Autodesk Inventor part; units mm, degrees
ref_plane "YZ Plane" through (0, 0, 0) normal (1, 0, 0) x (0, 1, 0)
ref_plane "XZ Plane" through (0, 0, 0) normal (0, 1, 0) x (-1, 0, 0)
ref_plane "XY Plane" through (0, 0, 0) normal (0, 0, 1) x (1, 0, 0)
sketch "Boceto1" plane through (0, 0, 0) normal (0, 1, 0) x (-1, 0, 0)
  line L0 (1.7308, 43.9183) -> (-63.2692, 43.9183)
  line L1 (-63.2692, 43.9183) -> (-63.2692, -61.0817)
  line L2 (-63.2692, -61.0817) -> (1.7308, -61.0817)
  line L3 (1.7308, -61.0817) -> (1.7308, 43.9183)
  point P0 (0, 0)
  dimension "d0" = 105
  dimension "d1" = 65
extrude "Extrusión1" add sketch "Boceto1" along normal blind 25
shell "Vaciado1" thickness 5 removed faces 1 at (19.9359, 25, -26.0817)
sketch "Boceto2" plane through (0, 25, 0) normal (0, 1, 0) x (1, 0, 0)
  line L0 (3.2692, 56.0817) -> (3.2692, -38.9183)
  line L1 (58.2692, 56.0817) -> (3.2692, 56.0817)
  line L2 (3.2692, 56.0817) -> (3.2692, -38.9183)
  line L3 (3.2692, -38.9183) -> (58.2692, -38.9183)
  line L4 (58.2692, -38.9183) -> (58.2692, 56.0817)
  point P0 (0, 0)
extrude "Extrusión2" add sketch "Boceto2" against normal blind 5
sketch "Boceto3" plane through (-1.7308, 0, 43.9183) normal (0, 0, 1) x (1, 0, 0)
  circle A0 centre (12.5, 12.5) radius 4.5
  line L0 (0, 0) -> (65, 0)
  line L1 (0, 0) -> (0, 25)
  point P0 (1.7308, 0)
  dimension "d12" = 9
  dimension "d13" = 12.5
  dimension "d14" = 12.5
extrude "Extrusión3" cut sketch "Boceto3" against normal blind 5
sketch "Boceto4" plane through (-1.7308, 0, 43.9183) normal (0, 0, 1) x (1, 0, 0)
  line L0 (60, 20) -> (5, 20)
  line L1 (60, 5) -> (5, 5)
  line L2 (29.5, 20) -> (35.5, 20)
  line L3 (35.5, 20) -> (35.5, 5)
  line L4 (35.5, 5) -> (29.5, 5)
  line L5 (29.5, 5) -> (29.5, 20)
  line L6 (0, 0) -> (0, 25)
  line L7 (65, 0) -> (65, 25)
  point P0 (1.7308, 0)
  point P1 (29.5, 12.5)
  point P2 (0, 12.5)
  dimension "d17" = 6
  dimension "d18" = 29.5
  dimension "d19" = 29.5
extrude "Extrusión4" cut sketch "Boceto4" against normal blind 5
sketch "Boceto5" plane through (-1.7308, 0, 43.9183) normal (0, 0, 1) x (1, 0, 0)
  line L0 (45, 16.5) -> (60, 16.5)
  line L1 (60, 16.5) -> (60, 8.5)
  line L2 (60, 8.5) -> (45, 8.5)
  line L3 (45, 8.5) -> (45, 16.5)
  line L4 (0, 25) -> (65, 25)
  line L5 (0, 0) -> (65, 0)
  line L6 (65, 0) -> (65, 25)
  point P0 (1.7308, 0)
  point P1 (52.5, 8.5)
  point P2 (52.5, 16.5)
  point P3 (60, 12.5)
  point P4 (45, 12.5)
  point P5 (65, 12.5)
  dimension "d22" = 8
  dimension "d23" = 15
  dimension "d24" = 8.5
  dimension "d25" = 8.5
  dimension "d26" = 5
extrude "Extrusión5" cut sketch "Boceto5" against normal blind 5
fillet "Empalme6" radius 2 1 edges at (-1.7308, 25, -8.5817)
fillet "Empalme7" radius 2 3 edges at (31.7692, 25, 43.9183) (-1.145, 24.4142, 43.9183) (-1.7308, 11.5, 43.9183)
fillet "Empalme8" radius 2 3 edges at (63.2692, 25, -9.5817) (63.2692, 24.4142, 43.3325) (63.2692, 11.5, 43.9183)
fillet "Empalme9" radius 2 5 edges at (30.7692, 25, -61.0817) (-1.145, 24.4142, -61.0817) (-1.7308, 11.5, -61.0817) (62.6834, 24.4142, -61.0817) (63.2692, 11.5, -61.0817)
fillet "Empalme10" radius 2 8 edges at (63.2692, 0, -8.5817) (62.6834, 0, -60.4959) (30.7692, 0, -61.0817) (-1.145, 0, -60.4959) (-1.7308, 0, -8.5817) (-1.145, 0, 43.3325) (30.7692, 0, 43.9183) (62.6834, 0, 43.3325)
properties part number "Lithium Battery"
CAD build for the part. Positions are in the model's coordinates, mm. A direction names the side the tool comes from. Give positions to 0.01 mm unless a question says otherwise; leave off trailing zeros. Loops run counter-clockwise (first coordinate to the right, second up) from the corner with the lowest first, then second, coordinate; pieces in that order, holes last. Notation, with made-up numbers: M 61,9.5 L 115,9.5 A25 cw 115,36.5 Z; hole C 61,-22 d4. An arc over 180 degrees is marked long. One line per question, with ' | ' between items. Start each with the question number.
1. Two-plate mould, pull along Y, no slides. Class faces 4 (the face through (63.269, 12, -8)), 5 (the face through (31, 20, -5)), 6 (the face through (31, 0, -8)): pulls with the +Y half, pulls with the -Y half, needs draft (parallel to the pull), parting line crosses it, or undercut.
2. Saw through at A-A on z = 14. Give the cut face in (x, y), plus the area to 3 significant figures.
3. Probe L1, parallel to X at y = 9.25, z = 20.5; L2, parallel to Y at x = 53.5, z = 10.5; L3, parallel to Z at x = 5, y = 19.5. List the from-to ranges inside material, lowest first. Write a range as from..to.
4. Saw through at B-B on y = 12.5. Give the cut face in (x, z), plus the area to 3 significant figures.
5. Saw through at C-C on x = 51. Give the cut face in (y, z), plus the area to 3 significant figures.
6. 3-axis set-ups, long thin cutter, end or side, ignore diameter. For faces 1 (the face through (62.7, 12.65, -60.48)), 2 (the face through (43, 12, 38.918)), 3 (the face through (33.769, 13, 41)): which of +Z, -Z, +X, -X, +Y, -Y reach the whole face in a straight line?
Result sheet:
1) face 4: needs draft | face 5: undercut | face 6: pulls with the -Y half
2) outline: M -1.73,2 A2 ccw 0.27,0 L 61.27,0 A2 ccw 63.27,2 L 63.27,23 A2 ccw 61.27,25 L 0.27,25 A2 ccw -1.73,23 Z; hole M 3.27,5 L 58.27,5 L 58.27,20 L 3.27,20 Z | area: 797 mm^2
3) L1: x = -1.73..3.27, 58.27..63.27 | L2: y = 0..5, 20..25 | L3: z = -61.08..-56.08, 38.92..43.92
4) outline: M -1.73,-59.08 A2 ccw 0.27,-61.08 L 61.27,-61.08 A2 ccw 63.27,-59.08 L 63.27,41.92 A2 ccw 61.27,43.92 L 58.27,43.92 L 58.27,-56.08 L 3.27,-56.08 L 3.27,38.92 L 6.27,38.92 L 6.27,43.92 L 0.27,43.92 A2 ccw -1.73,41.92 Z; M 15.27,38.92 L 27.77,38.92 L 27.77,43.92 L 15.27,43.92 Z; M 33.77,38.92 L 43.27,38.92 L 43.27,43.92 L 33.77,43.92 Z | area: 1,450 mm^2
5) outline: M 0,-59.08 A2 ccw 2,-61.08 L 23,-61.08 A2 ccw 25,-59.08 L 25,41.92 A2 ccw 23,43.92 L 16.5,43.92 L 16.5,38.92 L 20,38.92 L 20,-56.08 L 5,-56.08 L 5,38.92 L 8.5,38.92 L 8.5,43.92 L 2,43.92 A2 ccw 0,41.92 Z | area: 1,160 mm^2
6) face 1: -Z, +X, +Y, -Y | face 2: none | face 3: +Z
